Check sheet for the modelled part. Datum: model origin and axes. Units: mm. Face numbers are marked on the shaded views. A direction names the side the tool comes from. Round coordinates to 2 decimals unless told otherwise and drop trailing zeros. Write each loop counter-clockwise with the first axis right and the second up, starting at its lowest first coordinate (ties: lowest second). Pieces come first, ordered by that corner, then holes. Notation, with made-up numbers: (-9.5, 35) -> (29.5, 35) arc R14 cw to (29.5, 44) -> close; hole circle Ø3 at (34.25, 60). An arc over 180 degrees is marked (long way). Write item = value, one per line.
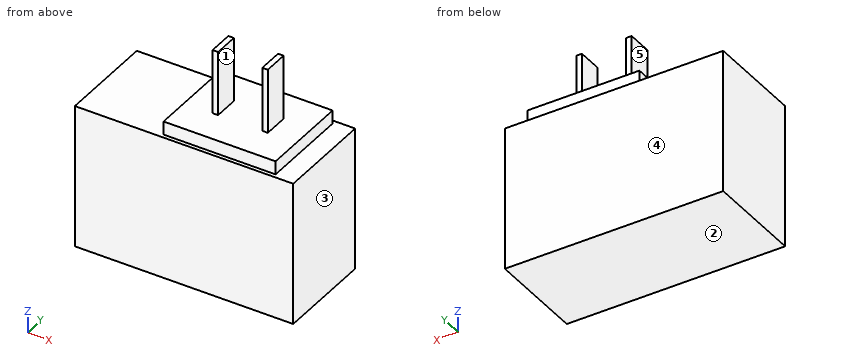
from build123d import *

# Parameters (mm, degrees)
SKETCH1_W           = 55.32
SKETCH1_H           = 24.84
BOSS_EXTRUDE1_DEPTH = 36.36
SKETCH2_W           = 28.38
SKETCH2_H           = 22.88
BOSS_EXTRUDE2_DEPTH = 3.39
SKETCH3_W           = 1.4
SKETCH3_H           = 6.32
BOSS_EXTRUDE3_DEPTH = 16.36


with BuildPart() as part:
    # Sketch1 → Boss-Extrude1 (new body)
    with BuildSketch(Plane.XY):
        Rectangle(SKETCH1_W, SKETCH1_H)
    extrude(amount=BOSS_EXTRUDE1_DEPTH)

    # Sketch2 → Boss-Extrude2 (add)
    with BuildSketch(Plane.XY.offset(36.36)):
        with Locations((8.38, 0)):
            Rectangle(SKETCH2_W, SKETCH2_H)
    extrude(amount=BOSS_EXTRUDE2_DEPTH)

    # Sketch3 → Boss-Extrude3 (add)
    with BuildSketch(Plane.XY.offset(39.75)):
        with Locations((14.68, 0)):
            Rectangle(SKETCH3_W, SKETCH3_H)
        with Locations((2.08, 0)):
            Rectangle(SKETCH3_W, SKETCH3_H)
    extrude(amount=BOSS_EXTRUDE3_DEPTH)


solid = part.part
(1) Material ranges on L1, parallel to X at y = -2, z = 54; L2, parallel to Z at x = -22, y = 9.25; L3, parallel to Z at x = 3, y = 7, recorded low to high. Write a range as [from, to].
Worked answers:
L1 = [1.38, 2.78], [13.98, 15.38]
L2 = [0, 36.36]
L3 = [0, 39.75]
(2) Sectioned sample at A-A on z = 43. Enter the section's corners in (x, y), then the cut area to 3 significant figures.
Worked answers:
outline = (1.38, -3.16) -> (2.78, -3.16) -> (2.78, 3.16) -> (1.38, 3.16) -> close; (13.98, -3.16) -> (15.38, -3.16) -> (15.38, 3.16) -> (13.98, 3.16) -> close
area = 17.7 mm²
(3) Sectioned sample at B-B on x = 8.5. Enter the section's corners in (y, z), then the cut area to 3 significant figures.
Worked answers:
outline = (-12.42, 0) -> (12.42, 0) -> (12.42, 36.36) -> (11.44, 36.36) -> (11.44, 39.75) -> (-11.44, 39.75) -> (-11.44, 36.36) -> (-12.42, 36.36) -> close
area = 981 mm²
(4) Release check for a two-part mould opening along X. For the marked faces 1, 2 and 3 record: pulls with the +X half, pulls with the -X half, needs draft (parallel to the pull), parting line crosses it, or undercut.
Worked answers:
face_1 = undercut
face_2 = needs draft
face_3 = pulls with the +X half
(5) Go/stop test with flat-tipped pins: P1, Ø1.1, axis at x = 14.5, z = 49.5, coming from the -Y side; P2, Ø2.5, axis at x = 4, z = 38, coming from the -Y side; P3, Ø1, axis at y = -0.5, z = 38.5, coming from the +X side. Record where each tip stops, or that it passes through.
Worked answers:
P1 = -3.16
P2 = -11.44
P3 = 22.57
(6) Sectioned sample at D-D on y = -1. Enter the section's corners in (x, z), then the cut area to 3 significant figures.
Worked answers:
outline = (-27.66, 0) -> (27.66, 0) -> (27.66, 36.36) -> (22.57, 36.36) -> (22.57, 39.75) -> (15.38, 39.75) -> (15.38, 56.11) -> (13.98, 56.11) -> (13.98, 39.75) -> (2.78, 39.75) -> (2.78, 56.11) -> (1.38, 56.11) -> (1.38, 39.75) -> (-5.81, 39.75) -> (-5.81, 36.36) -> (-27.66, 36.36) -> close
area = 2,150 mm²
(7) Access from +Z, -Z, +X, -X, +Y, -Y to the whole of each face (thin tool, end or side, straight path). Record for the marked faces 4 and 5.
Worked answers:
face_4 = +Z, -Z, +X, -X, +Y
face_5 = +Z, -X, +Y, -Y
(8) Sectioned sample at C-C on y = 6.75. Enter the section's corners in (x, z), then the cut area to 3 significant figures.
Worked answers:
outline = (-27.66, 0) -> (27.66, 0) -> (27.66, 36.36) -> (22.57, 36.36) -> (22.57, 39.75) -> (-5.81, 39.75) -> (-5.81, 36.36) -> (-27.66, 36.36) -> close
area = 2,110 mm²
